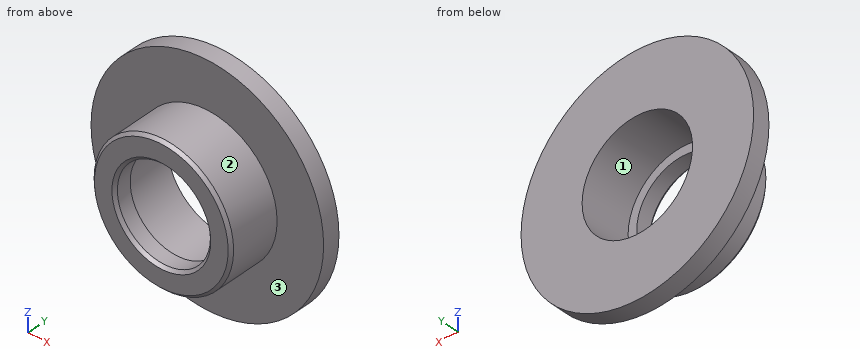
```python
from build123d import *

# Parameters (mm, degrees)
SMUSSO1_SIZE = 0.5


with BuildPart() as part:
    # Schizzo1 → Rivoluzione1 (revolve)
    with BuildSketch(Plane.XY):
        Polygon((9.5, 0), (20, 0), (20, -3), (12, -3), (12, -12), (8, -12), (8, -9), (9.5, -9), align=None)
    revolve(axis=Axis((0, -37.45263556, 0), (0, 1, 0)))

    # Smusso1
    smusso1_edges = [part.edges().sort_by_distance(p)[0] for p in [
        (-8, -12, 0),
        (-12, -12, 0),
    ]]
    chamfer(smusso1_edges, length=SMUSSO1_SIZE)


solid = part.part
```
For this review, take the finished solid that the model builds, in its own axes (mm). Face numbers are marked on the shaded views. Coordinates: 2 decimals unless noted, no trailing zeros. Loops run counter-clockwise (first coordinate to the right, second up) from the corner with the lowest first, then second, coordinate; pieces in that order, holes last. Notation, with made-up numbers: (73, 27) -> (121, 27) arc R31 ccw to (121, 54) -> close; hole circle Ø6 at (21.25, 73.25). An arc over 180 degrees is marked (long way). Return JSON: item names as keys, results as strings. Group by question number.
(1) For pin 1 Ø15 at (x, z) = (4, -0.5) entering from +Y; pin 2 Ø5 at (x, y) = (-8.5, -1.5) entering from -Z; pin 3 Ø5 at (y, z) = (-4, -8) entering from -X; pin 4 Ø6 at (x, y) = (5.5, -4) entering from +Z, all flat-tipped, find the tip position at first contact; note any pin that passes through.
(2) Consider section A-A, the plane z = 0. Give the boundary of the cut face in (x, y), plus the area to 4 significant figures.
(3) Consider section C-C, the plane y = -8.25. Give the boundary of the cut face in (x, z).
(4) Consider section B-B, the plane x = 0. Give the boundary of the cut face in (y, z), plus the area to 4 significant figures.
(5) Mouldability with a two-part tool opening along Z and no side actions: class the marked faces 1, 2 and 3 as pulls with the +Z half, pulls with the -Z half, needs draft (parallel to the pull), parting line crosses it, or undercut.
(6) To check wall thickness, follow L1, parallel to Z at x = 0, y = -4.25; L2, parallel to Z at x = 0, y = -10.15. State the ranges of each line that lie inside material, in increasing order.
(7) Consider section D-D, the plane z = 13. Give the boundary of the cut face in (x, y).
Results below:
{
 "1": {"pin 1": "stops at y = 0", "pin 2": "stops at z = -19.08", "pin 3": "stops at x = -19.17", "pin 4": "stops at z = 19.82"},
 "2": {"outline": "(-20, -3) -> (-12, -3) -> (-12, -11.5) -> (-11.5, -12) -> (-8.5, -12) -> (-8, -11.5) -> (-8, -9) -> (-9.5, -9) -> (-9.5, 0) -> (-20, 0) -> close; (8, -11.5) -> (8.5, -12) -> (11.5, -12) -> (12, -11.5) -> (12, -3) -> (20, -3) -> (20, 0) -> (9.5, 0) -> (9.5, -9) -> (8, -9) -> close", "area": "116.5 mm2"},
 "3": {"outline": "circle Ø24 at (0, 0); hole circle Ø19 at (0, 0)"},
 "4": {"outline": "(-12, -11.5) -> (-11.5, -12) -> (-3, -12) -> (-3, -20) -> (0, -20) -> (0, -9.5) -> (-9, -9.5) -> (-9, -8) -> (-11.5, -8) -> (-12, -8.5) -> close; (-12, 8.5) -> (-11.5, 8) -> (-9, 8) -> (-9, 9.5) -> (0, 9.5) -> (0, 20) -> (-3, 20) -> (-3, 12) -> (-11.5, 12) -> (-12, 11.5) -> close", "area": "116.5 mm2"},
 "5": {"face 1": "undercut", "face 2": "parting line crosses it", "face 3": "needs draft"},
 "6": {"L1": "z = -12 to -9.5, 9.5 to 12", "L2": "z = -12 to -8, 8 to 12"},
 "7": {"outline": "(-15.2, -3) -> (15.2, -3) -> (15.2, 0) -> (-15.2, 0) -> close"}
}
